Autodesk Inventor part; units mm, degrees
ref_plane "YZ Plane" through (0, 0, 0) normal (1, 0, 0) x (0, 1, 0)
ref_plane "XZ Plane" through (0, 0, 0) normal (0, 1, 0) x (-1, 0, 0)
ref_plane "XY Plane" through (0, 0, 0) normal (0, 0, 1) x (1, 0, 0)
sketch "Sketch1" plane through (0, 0, 0) normal (0, 0, 1) x (1, 0, 0)
  line L0 (-85, 15) -> (85, 15)
  line L1 (85, 15) -> (85, -15)
  line L2 (85, -15) -> (-85, -15)
  line L3 (-85, -15) -> (-85, 15)
  line L4 (85, -15) -> (-85, -15)
  line L5 (-85, -15) -> (-85, -36.3)
  line L6 (-85, -36.3) -> (85, -36.3)
  line L7 (85, -36.3) -> (85, -15)
  point P0 (0, 0)
  dimension "d0" = 30
  dimension "d1" = 170
  dimension "d2" = 85
  dimension "d3" = 15
  dimension "d34" = 21.3
  dimension "d35" = 170
extrude "Extrusion1" add sketch "Sketch1" along normal blind 10
sketch "Sketch2" plane through (0, 0, 10) normal (0, 0, 1) x (1, 0, 0)
  point P0 (0, 0)
  point P1 (-37.5, 0)
  point P2 (-12.5, 0)
  point P3 (12.5, 0)
  point P4 (37.5, 0)
  dimension "d30" = 25
  dimension "d31" = 25
  dimension "d32" = 25
  dimension "d33" = 12.5
hole "Hole1" at (-37.5, 0, 10) at (-12.5, 0, 10) at (12.5, 0, 10) at (37.5, 0, 10) direction (0, 0, -1) diameter 6.6 end through all counterbore diameter 11 counterbore depth 7
sketch "Sketch3" plane through (0, 0, 10) normal (0, 0, 1) x (1, 0, 0)
  point P0 (0, 0)
  point P1 (75, 0)
  point P2 (-75, 0)
  dimension "d16" = 150
  dimension "d17" = 75
hole "Hole2" at (75, 0, 10) at (-75, 0, 10) direction (0, 0, -1) diameter 3.242 end through all
equation "\"d35\" = d1"
properties part number "zStackJackAttach_piece1"
Model file for the job. Use its own axes, mm. A direction names the side the tool comes from. Round coordinates to 2 decimals unless told otherwise and drop trailing zeros. Write each loop counter-clockwise with the first axis right and the second up, starting at its lowest first coordinate (ties: lowest second). Pieces come first, ordered by that corner, then holes. Notation, with made-up numbers: (64, 23.5) - (83, 23.5) arc R14 cw to (83, 30.5) - close; hole circle Ø8 at (42.25, 31). An arc over 180 degrees is marked (long way). Use CSV: the item, a comma, the result in double quotes. Start each with the question number.
Item 1: Band-saw the part on C-C (x = -37.5). Write the cut outline in (y, z), and give its area (3 significant figures).
Item 2: Pin check, flat tip, straight feed: P1, Ø3.5, axis at x = -37, y = 2.5, coming from the +Z side. Stop position of the tip, or through.
Item 3: Tool access for faces 5 (the face through (34.23, 0.43, 1.48)), 6 (the face through (-7.13, 1.19, 6.45)): list every direction of +Z, -Z, +X, -X, +Y, -Y with a clear straight run to the whole face (end or side of a thin tool).
Item 4: Band-saw the part on B-B (z = 6.5). Write the cut outline in (x, y).
Item 5: Band-saw the part on A-A (x = -75). Write the cut outline in (y, z), and give its area (3 significant figures).
Item 6: Drill centre lines: L1, parallel to Y at x = 37.5, z = 7.5; L2, parallel to Y at x = 75, z = 6.25; L3, parallel to Z at x = 33.5, y = -2. Where is each one in solid material? Low to high. Write a range as [from, to].
Item 7: Two-plate mould, pull along Y, no slides. Class faces 1 (the face through (41, 0, 3)), 2 (the face through (-1, -36.3, 5)), 3 (the face through (-1, 15, 5)), 4 (the face through (-85, -11, 5)): released by +Y, released by -Y, zero draft, split by the parting line, or undercut.
Checked values:
1,outline,"(-36.3, 0) - (-3.3, 0) - (-3.3, 3) - (-5.5, 3) - (-5.5, 10) - (-36.3, 10) - close; (3.3, 0) - (15, 0) - (15, 10) - (5.5, 10) - (5.5, 3) - (3.3, 3) - close"
1,area,"416 mm²"
2,P1,"stops at z = 3"
3,face 5,"+Z, -Z"
3,face 6,"+Z"
4,outline,"(-85, -36.3) - (85, -36.3) - (85, 15) - (-85, 15) - close; hole circle Ø3.24 at (-75, 0); hole circle Ø11 at (-37.5, 0); hole circle Ø11 at (-12.5, 0); hole circle Ø11 at (12.5, 0); hole circle Ø11 at (37.5, 0); hole circle Ø3.24 at (75, 0)"
5,outline,"(-36.3, 0) - (-1.62, 0) - (-1.62, 10) - (-36.3, 10) - close; (1.62, 0) - (15, 0) - (15, 10) - (1.62, 10) - close"
5,area,"481 mm²"
6,L1,"y = [-36.3, -5.5], [5.5, 15]"
6,L2,"y = [-36.3, -1.62], [1.62, 15]"
6,L3,"z = [0, 3]"
7,face 1,"undercut"
7,face 2,"released by -Y"
7,face 3,"released by +Y"
7,face 4,"zero draft"
